```python
from build123d import *

# Parameters (mm, degrees)
SKETCH1_W           = 122.1
SKETCH1_H           = 197.8
BOSS_EXTRUDE2_DEPTH = 5
CUT_EXTRUDE1_DEPTH  = 5
SKETCH5_W           = 176.692600263
SKETCH5_H           = 67.834694549
CUT_EXTRUDE2_DEPTH  = 12
SKETCH6_W           = 148.50335492
SKETCH6_H           = 63.858757444
CUT_EXTRUDE3_DEPTH  = 19


with BuildPart() as part:
    # Sketch1 → Boss-Extrude2 (new body)
    with BuildSketch(Plane(origin=(0, 0, 0), x_dir=(1, 0, 0), z_dir=(0, 1, 0))):
        with Locations((61.05, 98.9)):
            Rectangle(SKETCH1_W, SKETCH1_H)
    extrude(amount=BOSS_EXTRUDE2_DEPTH)

    # Sketch3 → Cut-Extrude1 (cut)
    with BuildSketch(Plane(origin=(0, 5, 0), x_dir=(1, 0, 0), z_dir=(0, 1, 0))):
        with BuildLine():
            Line((10.5, 167.875007929), (10.5, 130.375007929))
            ThreePointArc((10.5, 130.375007929), (18, 122.875007929), (25.5, 130.375007929))
            Line((25.5, 130.375007929), (25.5, 167.875007929))
            ThreePointArc((25.5, 167.875007929), (18, 175.375007929), (10.5, 167.875007929))
        make_face()
        with BuildLine():
            ThreePointArc((111.6, 130.375007929), (104.1, 122.875007929), (96.6, 130.375007929))
            Line((96.6, 130.375007929), (96.6, 167.875007929))
            ThreePointArc((96.6, 167.875007929), (104.1, 175.375007929), (111.6, 167.875007929))
            Line((111.6, 167.875007929), (111.6, 130.375007929))
        make_face()
        with BuildLine():
            ThreePointArc((111.6, 49.721568021), (104.1, 42.221568021), (96.6, 49.721568021))
            Line((96.6, 49.721568021), (96.6, 87.221568021))
            ThreePointArc((96.6, 87.221568021), (104.1, 94.721568021), (111.6, 87.221568021))
            Line((111.6, 87.221568021), (111.6, 49.721568021))
        make_face()
        with BuildLine():
            Line((10.5, 87.221568021), (10.5, 49.721568021))
            ThreePointArc((10.5, 49.721568021), (18, 42.221568021), (25.5, 49.721568021))
            Line((25.5, 49.721568021), (25.5, 87.221568021))
            ThreePointArc((25.5, 87.221568021), (18, 94.721568021), (10.5, 87.221568021))
        make_face()
    extrude(amount=-CUT_EXTRUDE1_DEPTH, mode=Mode.SUBTRACT)

    # Sketch5 → Cut-Extrude2 (cut)
    with BuildSketch(Plane(origin=(0, 0, -197.8), x_dir=(-1, 0, 0), z_dir=(0, 0, -1))):
        with Locations((-46.708276043, -7.602787765)):
            Rectangle(SKETCH5_W, SKETCH5_H)
    extrude(amount=-CUT_EXTRUDE2_DEPTH, mode=Mode.SUBTRACT)

    # Sketch6 → Cut-Extrude3 (cut)
    with BuildSketch(Plane.XY):
        with Locations((68.056552209, 0.930489014)):
            Rectangle(SKETCH6_W, SKETCH6_H)
    extrude(amount=-CUT_EXTRUDE3_DEPTH, mode=Mode.SUBTRACT)


solid = part.part
```
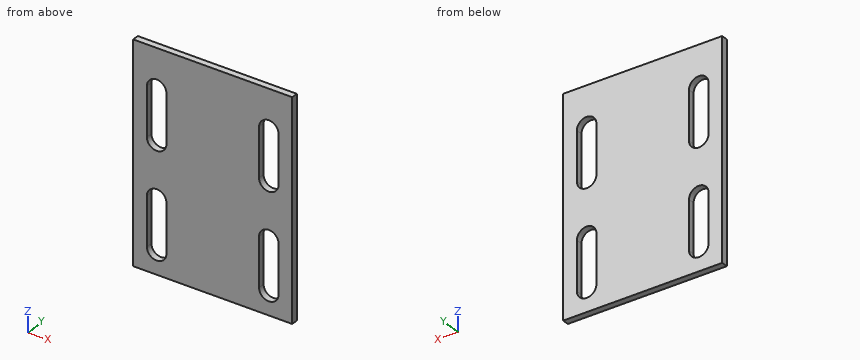
Geometry check sheet. Reference: the model listing, model coordinates, mm. Coordinates: 2 decimals unless noted, no trailing zeros. Order: outer loops, then holes, each group sorted by start corner. A loop starts at its lowest first (then second) coordinate and runs counter-clockwise, first axis right, second up. Notation, with made-up numbers: M 31,-38.75 L 75,-38.75 A27 ccw 75,-8.75 Z; hole C 34,-13 d1. An arc over 180 degrees is marked long. One line per question, with ' | ' between items. Start each with the question number.
Item 1: Material ranges on L1, parallel to X at y = 2.1, z = -84; L2, parallel to Z at x = 104, y = 2.7; L3, parallel to Z at x = 15, y = 3.6, recorded low to high. Write a range as [from, to].
Item 2: Cross-section at B-B on y = 2.5. Enter the section's corners in (x, z) (3 decimals), then the cut area to 3 significant figures.
Item 3: Cross-section at C-C on z = -147. Enter the section's corners in (x, y).
Item 4: Gauge pin test, flat end, axial feed: pin 1 (1.5 mm diameter, centred on x = 59.5, z = -133.5, fed in from -Y). Record the tip position at first contact, or that the pin passes through.
Item 5: Cross-section at A-A on x = 104.1. Enter the section's corners in (y, z) (3 decimals).
Findings:
1) L1: x = [0, 10.5], [25.5, 96.6], [111.6, 122.1] | L2: z = [-185.8, -175.37], [-122.88, -94.72], [-42.22, -19] | L3: z = [-185.8, -174.75], [-123.5, -94.1], [-42.85, -19]
2) outline: M 0,-185.8 L 122.1,-185.8 L 122.1,-19 L 0,-19 Z; hole M 10.5,-167.875 A7.5 ccw 25.5,-167.875 L 25.5,-130.375 A7.5 ccw 10.5,-130.375 Z; hole M 10.5,-87.222 A7.5 ccw 25.5,-87.222 L 25.5,-49.722 A7.5 ccw 10.5,-49.722 Z; hole M 96.6,-167.875 A7.5 ccw 111.6,-167.875 L 111.6,-130.375 A7.5 ccw 96.6,-130.375 Z; hole M 96.6,-87.222 A7.5 ccw 111.6,-87.222 L 111.6,-49.722 A7.5 ccw 96.6,-49.722 Z | area: 17,400 mm²
3) outline: M 0,0 L 10.5,0 L 10.5,5 L 0,5 Z; M 25.5,0 L 96.6,0 L 96.6,5 L 25.5,5 Z; M 111.6,0 L 122.1,0 L 122.1,5 L 111.6,5 Z
4) pin 1: stops at y = 0
5) outline: M 0,-185.8 L 5,-185.8 L 5,-175.375 L 0,-175.375 Z; M 0,-122.875 L 5,-122.875 L 5,-94.722 L 0,-94.722 Z; M 0,-42.222 L 5,-42.222 L 5,-19 L 0,-19 Z
